from build123d import *

# Parameters (mm, degrees)
SKETCH1_R           = 2.5
BOSS_EXTRUDE1_DEPTH = 6
BOSS_EXTRUDE2_START = -12.5
SKETCH2_W           = 6
SKETCH2_H           = 60
BOSS_EXTRUDE2_DEPTH = 60
BOSS_EXTRUDE3_START = -2
BOSS_EXTRUDE3_DEPTH = 6
BOSS_EXTRUDE4_START = -2
BOSS_EXTRUDE4_DEPTH = 6
SKETCH6_R           = 7.25
CUT_EXTRUDE1_DEPTH  = 86.546770833
CHAMFER3_SIZE       = 2


with BuildPart() as part:
    # Sketch1 → Boss-Extrude1 (new body)
    with BuildSketch(Plane(origin=(0, 0, 0), x_dir=(1, 0, 0), z_dir=(0, 1, 0))):
        with BuildLine():
            Line((-37.5, -20), (37.5, -20))
            ThreePointArc((37.5, -20), (41.035533906, -18.535533906), (42.5, -15))
            Line((42.5, -15), (42.5, 15))
            ThreePointArc((42.5, 15), (41.035533906, 18.535533906), (37.5, 20))
            Line((37.5, 20), (-37.5, 20))
            ThreePointArc((-37.5, 20), (-41.035533906, 18.535533906), (-42.5, 15))
            Line((-42.5, 15), (-42.5, -15))
            ThreePointArc((-42.5, -15), (-41.035533906, -18.535533906), (-37.5, -20))
        make_face()
        with Locations(Location((-15, 0, 0), (0, 0, 270))):
            Circle(SKETCH1_R, mode=Mode.SUBTRACT)
        with Locations(Location((15, 0, 0), (0, 0, 270))):
            Circle(SKETCH1_R, mode=Mode.SUBTRACT)
    extrude(amount=BOSS_EXTRUDE1_DEPTH)

    # Sketch2 → Boss-Extrude2 (add)
    with BuildSketch(Plane.ZY.offset(42.5).offset(BOSS_EXTRUDE2_START)):
        with Locations((-17, 36)):
            Rectangle(SKETCH2_W, SKETCH2_H)
    extrude(amount=-BOSS_EXTRUDE2_DEPTH)

    # Sketch4 → Boss-Extrude3 (add)
    with BuildSketch(Plane.ZY.offset(30).offset(BOSS_EXTRUDE3_START)):
        Polygon((16, 6), (-14, 44), (-14, 6), align=None)
    extrude(amount=-BOSS_EXTRUDE3_DEPTH)

    # Sketch5 → Boss-Extrude4 (add)
    with BuildSketch(Plane(origin=(30, 0, 0), x_dir=(0, 0, -1), z_dir=(1, 0, 0)).offset(BOSS_EXTRUDE4_START)):
        Polygon((-16, 6), (14, 44), (14, 6), align=None)
    extrude(amount=-BOSS_EXTRUDE4_DEPTH)

    # Sketch6 → Cut-Extrude1 (cut, through all)
    with BuildSketch(Plane.XY.offset(-14)):
        with Locations((0, 21)):
            Circle(SKETCH6_R)
    extrude(amount=-CUT_EXTRUDE1_DEPTH, mode=Mode.SUBTRACT)

    # Chamfer3
    chamfer3_edges = [part.edges().sort_by_distance(p)[0] for p in [
        (30, 66, -17),
        (-30, 66, -17),
    ]]
    chamfer(chamfer3_edges, length=CHAMFER3_SIZE)


solid = part.part
Geometry check sheet. Reference: the model listing, model coordinates, mm. A direction names the side the tool comes from. Round coordinates to 2 decimals unless told otherwise and drop trailing zeros. Order: outer loops, then holes, each group sorted by start corner. A loop starts at its lowest first (then second) coordinate and runs counter-clockwise, first axis right, second up. Notation, with made-up numbers: M 2.5,14 L 33.5,14 A21 cw 33.5,34 Z; hole C 32.25,73.25 d1. An arc over 180 degrees is marked long. Answer in a Markdown table with one row per item. Add a question column.
Item 1: Sectioned sample at D-D, the plane x = 25. Enter the section's corners in (y, z).
Item 2: Sectioned sample at C-C, the plane y = 15. Enter the section's corners in (x, z), plus the area to 3 significant figures.
Item 3: Draft check along Z on faces 1 (the face through (-41, 2.96, -18.57)), 2 (the face through (-17.44, 2.96, -0.54)), 3 (the face through (-30, 35, -17)). Enter one of: released by +Z, released by -Z, zero draft, split by the parting line, or undercut.
Item 4: Sectioned sample at B-B, the plane z = -1. Enter the section's corners in (x, y).
Item 5: Sectioned sample at A-A, the plane x = 15. Enter the section's corners in (y, z), plus the area to 3 significant figures.
Item 6: Material ranges on L1, parallel to X at y = 2.9, z = 0; L2, parallel to Y at x = 0, z = -16; L3, parallel to X at y = 14.5, z = -9.5, recorded low to high. Write a range as [from, to].
Item 7: Depth check by flat-ended pin: pin 1 Ø3 at (y, z) = (28.5, -17.5) entering from -X; pin 2 Ø3 at (y, z) = (38.5, -16) entering from +X; pin 3 Ø12 at (x, z) = (27.5, -1) entering from +Y. Enter the tip coordinate at first touch or a pass-through.
Item 8: Set-up check for faces 4 (the face through (-1, 6, 0)), 5 (the face through (0, 66, -17)), 6 (the face through (-28, 17, -6)): record each of +Z, -Z, +X, -X, +Y, -Y from which the full face is reachable in a straight line by a thin tool's end or side.
Filled in:
| question | item | result |
|---|---|---|
| 1 | outline | M 0,-20 L 66,-20 L 66,-14 L 44,-14 L 6,16 L 6,20 L 0,20 Z |
| 2 | outline | M -30,-20 L -4.07,-20 L -4.07,-14 L -22,-14 L -22,8.89 L -28,8.89 L -28,-14 L -30,-14 Z; M 4.07,-20 L 30,-20 L 30,-14 L 28,-14 L 28,8.89 L 22,8.89 L 22,-14 L 4.07,-14 Z |
| 2 | area | 586 mm² |
| 3 | face 1 | released by -Z |
| 3 | face 2 | undercut |
| 3 | face 3 | zero draft |
| 4 | outline | M -42.5,0 L -17.29,0 L -17.29,6 L -22,6 L -22,27.53 L -28,27.53 L -28,6 L -42.5,6 Z; M -12.71,0 L 12.71,0 L 12.71,6 L -12.71,6 Z; M 17.29,0 L 42.5,0 L 42.5,6 L 28,6 L 28,27.53 L 22,27.53 L 22,6 L 17.29,6 Z |
| 5 | outline | M 0,-20 L 66,-20 L 66,-14 L 6,-14 L 6,-2.5 L 0,-2.5 Z; M 0,2.5 L 6,2.5 L 6,20 L 0,20 Z |
| 5 | area | 570 mm² |
| 6 | L1 | x = [-42.5, -17.5], [-12.5, 12.5], [17.5, 42.5] |
| 6 | L2 | y = [0, 13.75], [28.25, 66] |
| 6 | L3 | x = [-28, -22], [22, 28] |
| 7 | pin 1 | stops at x = -30 |
| 7 | pin 2 | stops at x = 30 |
| 7 | pin 3 | stops at y = 35.13 |
| 8 | face 4 | +Z, +Y |
| 8 | face 5 | +Z, -Z, +X, -X, +Y |
| 8 | face 6 | +Z, -X, +Y |
